from build123d import *

# Parameters (mm, degrees)
SKETCH_1_R               = 30
SKETCH_1_R_2             = 28.6
EXTRUDE_1_DEPTH          = 80
PATTERN_CIRCULAR_1_COUNT = 8


with BuildPart() as part:
    # 스케치1 → 보스-돌출1 (new body)
    with BuildSketch(Plane(origin=(0, 0, 0), x_dir=(1, 0, 0), z_dir=(0, 1, 0))):
        with Locations(Location((0, 0, 0), (0, 0, 270))):
            Circle(SKETCH_1_R)
        with Locations(Location((0, 0, 0), (0, 0, 270))):
            Circle(SKETCH_1_R_2, mode=Mode.SUBTRACT)
    extrude(amount=EXTRUDE_1_DEPTH)

    # 스케치9 → M2 남비 머리 나사용 카운터보어1 (revolve, cut)
    with BuildSketch(Plane(origin=(-30, 5, 0), x_dir=(0, 0, 1), z_dir=(0, 1, 0))):
        Polygon((0, 0), (0, 10.721032743), (1.2, 10), (1.2, 1), (2.5, 1), (2.5, 0), align=None)
    hole_wizard_m2_1 = revolve(axis=Axis((-36.35, 5, 0), (1, 0, 0)), mode=Mode.SUBTRACT)

    # 원형 패턴1: M2 남비 머리 나사용 카운터보어1 ×8 about axis
    pattern_circular_1_axis = Axis((0, 0, 0), (0, 1, 0))
    for i in range(1, PATTERN_CIRCULAR_1_COUNT):
        add(hole_wizard_m2_1.rotate(pattern_circular_1_axis, i * 360 / PATTERN_CIRCULAR_1_COUNT), mode=Mode.SUBTRACT)


solid = part.part
The model under review builds one solid part; all positions refer to its coordinate system, in mm. A direction names the side the tool comes from. Coordinates: 2 decimals unless noted, no trailing zeros. Write each loop counter-clockwise with the first axis right and the second up, starting at its lowest first coordinate (ties: lowest second). Pieces come first, ordered by that corner, then holes. Notation, with made-up numbers: M 28,36.5 L 65,36.5 A18 ccw 65,65.5 Z; hole C -17.75,51.25 d1. An arc over 180 degrees is marked long. Put each result on its own line as item: value.
1) Add section D-D on x = 15.5. Give the boundary of the cut face in (y, z), then the cut area to 3 significant figures.
Computed:
outline: M 0,-25.69 L 80,-25.69 L 80,-24.04 L 0,-24.04 Z; M 0,24.04 L 80,24.04 L 80,25.69 L 0,25.69 Z
area: 264 mm2
2) Add section B-B on x = 0. Give the boundary of the cut face in (y, z).
Computed:
outline: M 0,-30 L 2.5,-30 L 2.5,-29 L 3.8,-29 L 3.8,-28.6 L 0,-28.6 Z; M 0,28.6 L 3.8,28.6 L 3.8,29 L 2.5,29 L 2.5,30 L 0,30 Z; M 6.2,-29 L 7.5,-29 L 7.5,-30 L 80,-30 L 80,-28.6 L 6.2,-28.6 Z; M 6.2,28.6 L 80,28.6 L 80,30 L 7.5,30 L 7.5,29 L 6.2,29 Z
3) Draft analysis for pull direction Z (two halves, no side actions). For faces 1 (the flat face through (-11, 80, 27)), 2 (the flat face through (1, 6, 29)), 3 (the cylindrical face through (22.55, 4.25, 19.18)), state which applies: released by +Z, released by -Z, zero draft, split by the parting line, or undercut.
Computed:
face 1: zero draft
face 2: released by +Z
face 3: undercut
4) Wall thickness on probe 1 along Z at (x, y) = (0, 42); probe 2 along Y at (x, z) = (-20, -21.5); probe 3 along X at (y, z) = (71, -12.5): over which ranges is each line inside the solid? List them lowest first. Write a range as [from, to].
Computed:
probe 1: z = [-30, -28.6], [28.6, 30]
probe 2: y = [0, 2.74], [7.26, 80]
probe 3: x = [-27.27, -25.72], [25.72, 27.27]
5) Add section A-A on z = 0. Give the boundary of the cut face in (x, y).
Computed:
outline: M -30,0 L -28.6,0 L -28.6,3.8 L -29,3.8 L -29,2.5 L -30,2.5 Z; M -30,7.5 L -29,7.5 L -29,6.2 L -28.6,6.2 L -28.6,80 L -30,80 Z; M 28.6,0 L 30,0 L 30,2.5 L 29,2.5 L 29,3.8 L 28.6,3.8 Z; M 28.6,6.2 L 29,6.2 L 29,7.5 L 30,7.5 L 30,80 L 28.6,80 Z
6) Add section C-C on y = 37. Give the boundary of the cut face in (x, z).
Computed:
outline: C 0,0 d60; hole C 0,0 d57.2
7) Clearance check with flat-ended pins moving along their axes: pin 1 Ø1.5 at (x, y) = (20.5, 41.5) entering from +Z; pin 2 Ø10 at (x, z) = (7, 23) entering from +Y; pin 3 Ø3 at (y, z) = (5, 0) entering from -X; pin 4 Ø4 at (x, y) = (0, 5) entering from -Z. State where each tip first meets the part, or that it passes through.
Computed:
pin 1: stops at z = 22.58
pin 2: stops at y = 80
pin 3: stops at x = -29
pin 4: stops at z = -29
8) For faces 4 (the cylindrical face through (-19.55, 4.64, 21.17)), 5 (the cylindrical face through (29.507, 4.249, -2.385)), 6 (the cylindrical face through (-2.385, 4.249, -29.507)), list the 3-axis set-ups (+Z, -Z, +X, -X, +Y, -Y) from which the entire face can be reached by the end or side of a thin tool; tool diameter is ignored.
Computed:
face 4: none
face 5: +X
face 6: -Z
